The figure shows three views and two pictorial views of one solid part (mm, origin at its lowest corner). Answer the questions. Give positions to 0.01 mm unless a question says otherwise; leave off trailing zeros. Write each loop counter-clockwise with the first axis right and the second up, starting at its lowest first coordinate (ties: lowest second). Pieces come first, ordered by that corner, then holes. Notation, with made-up numbers: (70.25, -38.5) -> (75.25, -38.5) arc R24 ccw to (75.25, -7.5) -> close; hole circle Ø5 at (59, -23.5). An arc over 180 degrees is marked (long way). Write each question's results on one line, items separated by ' | '. Start each with the question number.
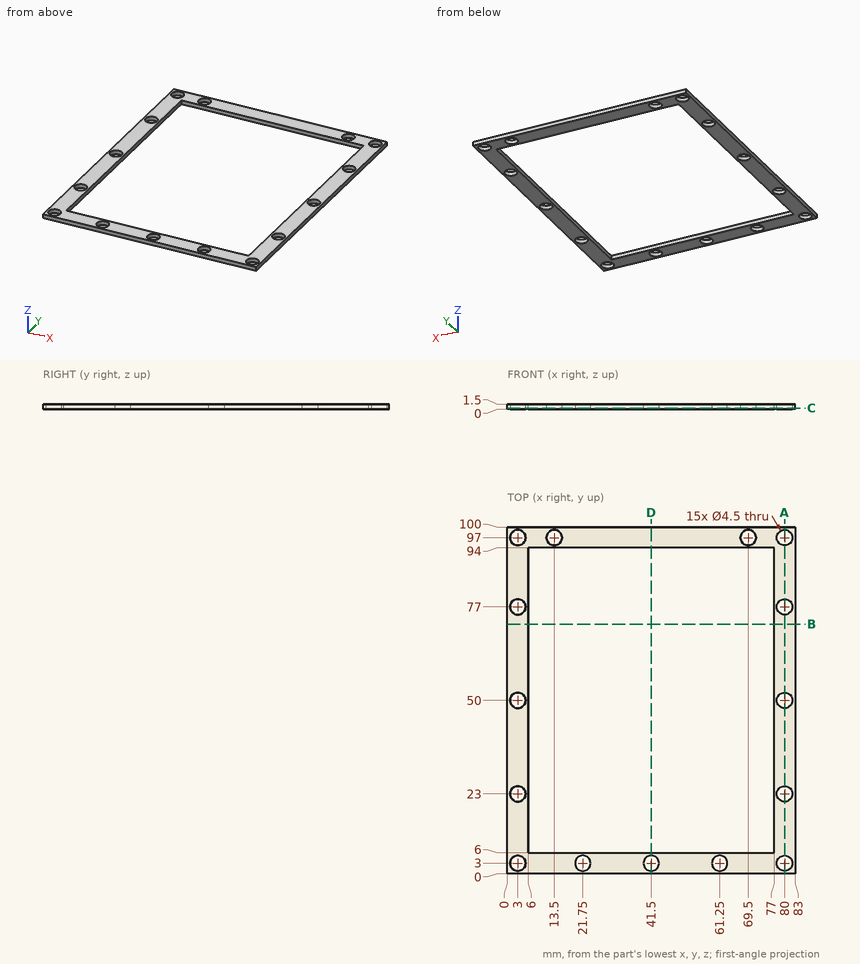
1. Section B-B (y = 72) is taken. Write down the section's boundary in (x, z), then the cut area to 3 significant figures.
2. Consider probe 1 along Y at (x, z) = (3, 1.15); probe 2 along Y at (x, z) = (76, 1.1); probe 3 along X at (y, z) = (90.5, 1.45). Determine where each line is inside the solid, lowest interval first. Write a range as [from, to].
3. Section C-C (z = 0.3) is taken. Give the number of separate pieces and of enclosed holes in the cut face, then the cut area to 3 significant figures.
4. Section A-A (x = 80) is taken. Write down the section's boundary in (y, z), then the cut area to 3 significant figures.
5. Section D-D (x = 41.5) is taken. Write down the section's boundary in (y, z).
Results:
1) outline: (0, 0) -> (6, 0) -> (6, 1.5) -> (0, 1.5) -> close; (77, 0) -> (83, 0) -> (83, 1.5) -> (77, 1.5) -> close | area: 18.0 mm²
2) probe 1: y = [0, 0.75], [5.25, 20.75], [25.25, 47.75], [52.25, 74.75], [79.25, 94.75], [99.25, 100] | probe 2: y = [0, 6], [94, 100] | probe 3: x = [0, 6], [77, 83]
3) separate pieces: 1 | enclosed holes: 16 | area: 1,810 mm²
4) outline: (0, 0) -> (0.75, 0) -> (0.75, 1.5) -> (0, 1.5) -> close; (5.25, 0) -> (20.75, 0) -> (20.75, 1.5) -> (5.25, 1.5) -> close; (25.25, 0) -> (47.75, 0) -> (47.75, 1.5) -> (25.25, 1.5) -> close; (52.25, 0) -> (74.75, 0) -> (74.75, 1.5) -> (52.25, 1.5) -> close; (79.25, 0) -> (94.75, 0) -> (94.75, 1.5) -> (79.25, 1.5) -> close; (99.25, 0) -> (100, 0) -> (100, 1.5) -> (99.25, 1.5) -> close | area: 116 mm²
5) outline: (0, 0) -> (0.75, 0) -> (0.75, 1.5) -> (0, 1.5) -> close; (5.25, 0) -> (6, 0) -> (6, 1.5) -> (5.25, 1.5) -> close; (94, 0) -> (100, 0) -> (100, 1.5) -> (94, 1.5) -> close
